Design review of the part built by this model. Coordinates are the model's own, in mm. A direction names the side the tool comes from. Round coordinates to 2 decimals unless told otherwise and drop trailing zeros. Order: outer loops, then holes, each group sorted by start corner. A loop starts at its lowest first (then second) coordinate and runs counter-clockwise, first axis right, second up. Notation, with made-up numbers: M 16.5,-38.75 L 36.5,-38.75 A14 cw 36.5,-19.75 Z; hole C -13.75,-11 d7. An arc over 180 degrees is marked long. Write item = value, one per line. Start each with the question number.
```python
from build123d import *

# Parameters (mm, degrees)
SALIENTE_EXTRUIR1_DEPTH = 100
CROQUIS2_R              = 2.5
CORTAR_EXTRUIR1_DEPTH   = 10
CROQUIS3_W              = 8
CROQUIS3_H              = 40
CORTAR_EXTRUIR2_DEPTH   = 201


with BuildPart() as part:
    # Croquis1 → Saliente-Extruir1 (new body, symmetric)
    with BuildSketch(Plane.XY):
        Polygon((-27, 20), (-27, -20), (27, -20), (27, 20), (25, 20), (25, -18), (-25, -18), (-25, 20), align=None)
    extrude(amount=SALIENTE_EXTRUIR1_DEPTH, both=True)

    # Croquis2 → Cortar-Extruir1 (cut)
    with BuildSketch(Plane(origin=(27, 0, 0), x_dir=(0, 0, -1), z_dir=(1, 0, 0))):
        with Locations((-55.4, 0)):
            Circle(CROQUIS2_R)
        with Locations((-22.62, 0)):
            Circle(CROQUIS2_R)
        with Locations((10.16, 0)):
            Circle(CROQUIS2_R)
        with Locations((42.94, 0)):
            Circle(CROQUIS2_R)
        with Locations((75.72, 0)):
            Circle(CROQUIS2_R)
    extrude(amount=-CORTAR_EXTRUIR1_DEPTH, mode=Mode.SUBTRACT)

    # Croquis3 → Cortar-Extruir2 (cut, through all)
    with BuildSketch(Plane.XY.offset(100)):
        with Locations((-23, 0)):
            Rectangle(CROQUIS3_W, CROQUIS3_H)
    extrude(amount=-CORTAR_EXTRUIR2_DEPTH, mode=Mode.SUBTRACT)


solid = part.part
```
(1) Consider section C-C, the plane z = -85. Write out the cut boundary in (x, y), then the cut area to 3 significant figures.
(2) Consider section A-A, the plane z = 55.4. Write out the cut boundary in (x, y), then the cut area to 3 significant figures.
(3) For line 1 along Y through (x, z) = (26.2, -42.94); line 2 along X through (y, z) = (7, -23); line 3 along Y through (x, z) = (-9, 23), list the stretches that pass through material, from the lowest coordinate up. Write a range as [from, to].
(4) Consider section D-D, the plane y = 7.5. Write out the cut boundary in (x, z), then the cut area to 3 significant figures.
(5) Insertion check: pin 1 (3 mm diameter, centred on y = -1, z = -41.5, fed in from -X); pin 2 (13 mm diameter, centred on x = 12.5, z = 44, fed in from +Y); pin 3 (6 mm diameter, centred on y = 0, z = 22.62, fed in from +X). Each pin has a flat end and moves straight along its axis. Give the tip position at first contact, or say it passes through.
(6) Consider section B-B, the plane y = 0. Write out the cut boundary in (x, z), then the cut area to 3 significant figures.
(7) For faces 4 (the face through (26.01, -0.96, -45.25)), 5 (the face through (25, 1, 1)), list the 3-axis set-ups (+Z, -Z, +X, -X, +Y, -Y) from which the entire face can be reached by the end or side of a thin tool; tool diameter is ignored.
(8) Draft analysis for pull direction Y (two halves, no side actions). For faces 1 (the face through (26.01, -0.96, 53.09)), 2 (the face through (3, -18, 1)), 3 (the face through (14, -19, -100)), state which applies: pulls with the +Y half, pulls with the -Y half, needs draft (parallel to the pull), parting line crosses it, or undercut.
Completed:
q1.outline = M -19,-20 L 27,-20 L 27,20 L 25,20 L 25,-18 L -19,-18 Z
q1.area = 168 mm2
q2.outline = M -19,-20 L 27,-20 L 27,-2.5 L 25,-2.5 L 25,-18 L -19,-18 Z; M 25,2.5 L 27,2.5 L 27,20 L 25,20 Z
q2.area = 158 mm2
q3.line_1 = [-20, -2.5], [2.5, 20]
q3.line_2 = [25, 27]
q3.line_3 = [-20, -18]
q4.outline = M 25,-100 L 27,-100 L 27,100 L 25,100 Z
q4.area = 400 mm2
q5.pin_1 = 25
q5.pin_2 = -18
q5.pin_3 = 27
q6.outline = M 25,-100 L 27,-100 L 27,-78.22 L 25,-78.22 Z; M 25,-73.22 L 27,-73.22 L 27,-45.44 L 25,-45.44 Z; M 25,-40.44 L 27,-40.44 L 27,-12.66 L 25,-12.66 Z; M 25,-7.66 L 27,-7.66 L 27,20.12 L 25,20.12 Z; M 25,25.12 L 27,25.12 L 27,52.9 L 25,52.9 Z; M 25,57.9 L 27,57.9 L 27,100 L 25,100 Z
q6.area = 350 mm2
q7.face_4 = +X, -X
q7.face_5 = +Z, -Z, -X, +Y
q8.face_1 = undercut
q8.face_2 = pulls with the +Y half
q8.face_3 = needs draft
